Part model, mm, in its own coordinate system. Face numbers are marked on the shaded views. A direction names the side the tool comes from. Coordinates: 2 decimals unless noted, no trailing zeros. Answer as a JSON object with one key per item and string values. Group by question number.
1. Mould opens along X. For the marked faces 1, 2, 3 and 4 say: released by +X, released by -X, zero draft, split by the parting line, or undercut.
2. 3-axis set-ups, long thin cutter, end or side, ignore diameter. For the marked faces 5, 6, 7 and 8: which of +Z, -Z, +X, -X, +Y, -Y reach the whole face in a straight line?
3. Drop flat-ended pins along their axis: pin 1 Ø2 at (x, y) = (-8.5, 5) entering from -Z; pin 2 Ø6 at (x, y) = (0, 40.5) entering from -Z; pin 3 Ø3.5 at (y, z) = (39, -2.5) entering from +X. Give the stop position or say it passes through.
4. Drill centre lines: L1, parallel to Y at x = -3.25, z = -24; L2, parallel to Z at x = -10, y = 38; L3, parallel to Z at x = -10.5, y = 42.5. Where is each one in solid material? Low to high.
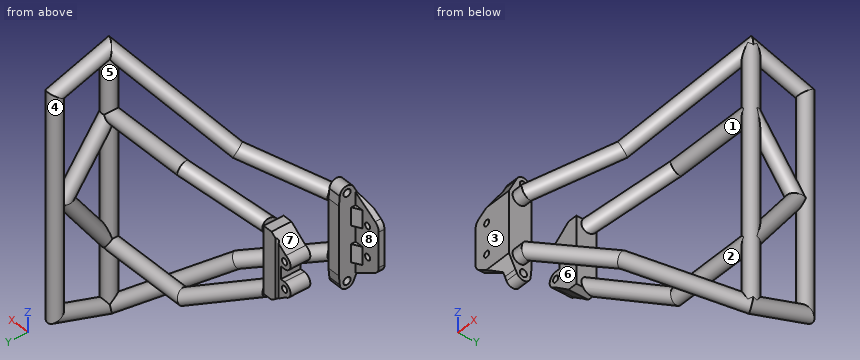
from build123d import *

# Parameters (mm, degrees)
SKETCH1_R               = 1.7
BOSS_EXTRUDE1_DEPTH     = 12.5
SKETCH2_W               = 15.5
SKETCH2_H               = 9.3
CUT_EXTRUDE1_DEPTH      = 55.465585465
BOSS_EXTRUDE2_DEPTH     = 7
CUT_EXTRUDE2_START      = -7
CUT_EXTRUDE2_DEPTH      = 15.157895
CUT_EXTRUDE3_REACH      = 36.358
SKETCH6_R               = 2
BOSS_EXTRUDE3_DEPTH     = 15
CUT_EXTRUDE4_REACH      = 39.104
SKETCH8_W               = 4.5
SKETCH8_H               = 10
SWEEP1_PROFILE_R        = 4
SWEEP4_PROFILE_R        = 4
SWEEP5_PROFILE_R        = 4
SKETCH107_W             = 7.357095587
SKETCH107_H             = 45.138164382
CUT_EXTRUDE5_DEPTH      = 10
CUT_EXTRUDE5_DEPTH_BACK = 10
SKETCH106_R             = 1.75
BOSS_EXTRUDE4_DEPTH     = 5.5
CUT_EXTRUDE6_DEPTH      = 163.309191318


with BuildPart() as part:
    # Sketch1 → Boss-Extrude1 (new body)
    with BuildSketch(Plane(origin=(0, 0, 0), x_dir=(1, 0, 0), z_dir=(0, 1, 0))):
        with BuildLine():
            Line((0, 24), (0, -24))
            Line((0, -24), (-7, -24))
            Line((-7, -24), (-7, -22))
            Line((-7, -22), (-20.11281029, -13.963116274))
            ThreePointArc((-20.11281029, -13.963116274), (-21.862570999, -12.143053785), (-22.5, -9.700110012))
            Line((-22.5, -9.700110012), (-22.5, 9.700110012))
            ThreePointArc((-22.5, 9.700110012), (-21.862570999, 12.143053785), (-20.11281029, 13.963116274))
            Line((-20.11281029, 13.963116274), (-7, 22))
            Line((-7, 22), (-7, 24))
            Line((-7, 24), (0, 24))
        make_face()
        with Locations(Location((-15, -8.5, 0), (0, 0, 270))):
            Circle(SKETCH1_R, mode=Mode.SUBTRACT)
        with Locations(Location((-15, 8.5, 0), (0, 0, 90))):
            Circle(SKETCH1_R, mode=Mode.SUBTRACT)
    extrude(amount=BOSS_EXTRUDE1_DEPTH)

    # Sketch2 → Cut-Extrude1 (cut, through all)
    with BuildSketch(Plane.XY.offset(24)):
        with Locations((-14.75, 7.85)):
            Rectangle(SKETCH2_W, SKETCH2_H)
    extrude(amount=-CUT_EXTRUDE1_DEPTH, mode=Mode.SUBTRACT)

    # Sketch4 → Boss-Extrude2 (add)
    with BuildSketch(Plane.ZY.offset(7)):
        with BuildLine():
            Line((25.797906634, 4.426831695), (24, 3.522181259))
            Line((24, 3.522181259), (24, 12.018504252))
            Line((24, 12.018504252), (24.38342286, 11.981580956))
            ThreePointArc((24.38342286, 11.981580956), (27.931680136, 8.736132671), (25.797906634, 4.426831695))
        make_face()
        with BuildLine():
            Line((-24, 3.522181259), (-24, 12.018504252))
            Line((-24, 12.018504252), (-24.38342286, 11.981580956))
            ThreePointArc((-24.38342286, 11.981580956), (-27.931680136, 8.736132671), (-25.797906634, 4.426831695))
            Line((-25.797906634, 4.426831695), (-24, 3.522181259))
        make_face()
    extrude(amount=-BOSS_EXTRUDE2_DEPTH)

    # Sketch5 → Cut-Extrude2 (cut)
    with BuildSketch(Plane.ZY.offset(7).offset(CUT_EXTRUDE2_START)):
        Polygon((24, 3.522181259), (17, 0), (24, 0), align=None)
        Polygon((24, 12.018504252), (19, 12.5), (24, 12.5), align=None)
        Polygon((-24, 12.5), (-24, 12.018504252), (-19, 12.5), align=None)
        Polygon((-24, 0), (-24, 3.522181259), (-17, 0), align=None)
    extrude(amount=CUT_EXTRUDE2_DEPTH, mode=Mode.SUBTRACT)

    # Sketch6 → Cut-Extrude3 (cut, up to next)
    with BuildSketch(Plane.ZY.offset(7), mode=Mode.PRIVATE) as cut_extrude3_sk1:
        with Locations((-24, 8)):
            Circle(SKETCH6_R)
    cut_extrude3_tool1 = extrude(cut_extrude3_sk1.sketch, amount=-CUT_EXTRUDE3_REACH, mode=Mode.PRIVATE) & part.part
    # Sketch6 → Cut-Extrude3 (cut, up to next)
    with BuildSketch(Plane.ZY.offset(7), mode=Mode.PRIVATE) as cut_extrude3_sk2:
        with Locations((24, 8)):
            Circle(SKETCH6_R)
    cut_extrude3_tool2 = extrude(cut_extrude3_sk2.sketch, amount=-CUT_EXTRUDE3_REACH, mode=Mode.PRIVATE) & part.part
    add(cut_extrude3_tool1.solids().sort_by_distance((-7, 8, -24))[0], mode=Mode.SUBTRACT)
    add(cut_extrude3_tool2.solids().sort_by_distance((-7, 8, 24))[0], mode=Mode.SUBTRACT)

    # Sketch7 → Boss-Extrude3 (add, symmetric)
    with BuildSketch(Plane.XY):
        Polygon((-11.5, 3.2), (-7, 3.2), (-7, 5.7), align=None)
    extrude(amount=BOSS_EXTRUDE3_DEPTH, both=True)

    # Cut-Extrude4: up to this face of the body (flat: up to its plane)
    cut_extrude4_end = Plane(part.part.faces().sort_by_distance((-9.25, 4.45, 0))[0])
    # Sketch8 → Cut-Extrude4 (cut, up to the picked face)
    with BuildSketch(Plane(origin=(0, 3.2, 0), x_dir=(1, 0, 0), z_dir=(0, 1, 0)), mode=Mode.PRIVATE) as cut_extrude4_sk1:
        with Locations((-9.25, 0)):
            Rectangle(SKETCH8_W, SKETCH8_H)
    cut_extrude4_tool1 = split(extrude(cut_extrude4_sk1.sketch, amount=CUT_EXTRUDE4_REACH, mode=Mode.PRIVATE), bisect_by=cut_extrude4_end, keep=Keep.BOTH, mode=Mode.PRIVATE)
    add(cut_extrude4_tool1.solids().sort_by(Axis((-9.25, 3.2, 0), (0, 1, 0)))[0], mode=Mode.SUBTRACT)

    # Sweep1: sweep along a curve in space
    with BuildLine() as sweep1_path:
        Line((0, 6, 16), (5, 6, 16))
        Line((5, 6, 16), (40, 30, 30))
        Line((40, 30, 30), (90, 60, 70))
        Line((90, 60, 70), (90, 90, 60))
        Line((90, 90, 60), (90, 90, -60))
        Line((90, 90, -60), (90, 60, -70))
        Line((40, 30, -30), (90, 60, -70))
        Line((5, 6, -16), (40, 30, -30))
        Line((0, 6, -16), (5, 6, -16))
    # Sweep1 profile (on start of the path) → Sweep1 (sweep)
    with BuildSketch(Plane(origin=(0, 6, 16), x_dir=(0, 0, 1), z_dir=(1, 0, 0))):
        Circle(SWEEP1_PROFILE_R)
    sweep(path=sweep1_path.line, transition=Transition.RIGHT)



with BuildPart() as body_2:
    # Sweep4: sweep along a curve in space
    with BuildLine() as sweep4_path:
        Line((40, 60, -35), (0, 40, -15))
        Line((90, 60, -35), (40, 60, -35))
        Line((90, 60, -35), (90, 60, 35))
        Line((90, 60, 35), (40, 60, 35))
        Line((40, 60, 35), (0, 40, 15))
    # Sweep4 profile (on start of the path) → Sweep4 (sweep)
    with BuildSketch(Plane(origin=(0, 40, 15), x_dir=(-0.4472135954999578, 0, 0.894427190999916), z_dir=(0.816496580927726, 0.40824829046386285, 0.40824829046386285))):
        Circle(SWEEP4_PROFILE_R)
    sweep(path=sweep4_path.line, transition=Transition.RIGHT)


with BuildPart() as part_1:
    add(part.part)

    add(body_2.part)  # Sweep5 merges body 2
    # Sweep5: sweep along a curve in space
    with BuildLine() as sweep5_path:
        Line((90, 60, -70), (90, 60, -35))
        Line((90, 60, -35), (90, 85, 0))
        Line((90, 85, 0), (90, 60, 35))
        Line((90, 60, 35), (90, 60, 70))
    # Sweep5 profile (on start of the path) → Sweep5 (sweep)
    with BuildSketch(Plane(origin=(90, 60, -70), x_dir=(1, 0, 0), z_dir=(0, 0, 1))):
        Circle(SWEEP5_PROFILE_R)
    sweep(path=sweep5_path.line, transition=Transition.RIGHT)

    # Sketch107 → Cut-Extrude5 (cut, two sides)
    with BuildSketch(Plane(origin=(0, 40, 0), x_dir=(1, 0, 0), z_dir=(0, 1, 0))) as cut_extrude5_sk:
        with Locations((-0.178547794, 0.105399285)):
            Rectangle(SKETCH107_W, SKETCH107_H)
    extrude(amount=CUT_EXTRUDE5_DEPTH, mode=Mode.SUBTRACT)
    extrude(cut_extrude5_sk.sketch, amount=-CUT_EXTRUDE5_DEPTH_BACK, mode=Mode.SUBTRACT)

    # Sketch106 → Boss-Extrude4 (add, symmetric)
    with BuildSketch(Plane(origin=(0, 40, 0), x_dir=(1, 0, 0), z_dir=(0, 1, 0))):
        with BuildLine():
            Line((-1.788854382, -18.577708764), (-11.388819442, -11.4))
            ThreePointArc((-11.388819442, -11.4), (-14.474921383, -7.052786405), (-10.5, -3.5))
            Line((-10.5, -3.5), (-8, -3.5))
            Line((-8, -3.5), (-8, 3.5))
            Line((-8, 3.5), (-10.5, 3.5))
            ThreePointArc((-10.5, 3.5), (-14.474921383, 7.052786405), (-11.388819442, 11.4))
            Line((-11.388819442, 11.4), (-1.788854382, 18.577708764))
            Line((-1.788854382, 18.577708764), (3.501145618, 18.577708764))
            Line((3.501145618, 18.577708764), (3.501145618, -18.577708764))
            Line((3.501145618, -18.577708764), (-1.788854382, -18.577708764))
        make_face()
        with Locations(Location((-10.5, 7.5, 0), (0, 0, 180))):
            Circle(SKETCH106_R, mode=Mode.SUBTRACT)
        with Locations(Location((-10.5, -7.5, 0), (0, 0, 180))):
            Circle(SKETCH106_R, mode=Mode.SUBTRACT)
    extrude(amount=BOSS_EXTRUDE4_DEPTH, both=True)

    # Sketch108 → Cut-Extrude6 (cut, through all)
    with BuildSketch(Plane(origin=(0, 0, -18.577708764), x_dir=(-1, 0, 0), z_dir=(0, 0, -1))):
        with BuildLine():
            Line((4.6, 45.5), (6.4, 45.5))
            ThreePointArc((6.4, 45.5), (5.5, 44.6), (4.6, 45.5))
        make_face()
    extrude(amount=-CUT_EXTRUDE6_DEPTH, mode=Mode.SUBTRACT)


solid = part_1.part
Outcome:
{
 "1": {"face 1": "undercut", "face 2": "undercut", "face 3": "zero draft", "face 4": "split by the parting line"},
 "2": {"face 5": "none", "face 6": "+Z, -Z, +X, -X", "face 7": "+Z, -X, +Y", "face 8": "-X"},
 "3": {"pin 1": "stops at z = -15", "pin 2": "stops at z = -18.58", "pin 3": "stops at x = 3.5"},
 "4": {"L1": "y = 3.52 to 6, 10 to 12.02", "L2": "z = -12.44 to -9.18, -5.82 to -3.5, 3.5 to 5.82, 9.18 to 12.44", "L3": "z = -12.06 to -9.25, -5.75 to -3.5, 3.5 to 5.75, 9.25 to 12.06"}
}
